The model under review builds one solid part; all positions refer to its coordinate system, in mm. Round coordinates to 2 decimals unless told otherwise and drop trailing zeros. Loops run counter-clockwise (first coordinate to the right, second up) from the corner with the lowest first, then second, coordinate; pieces in that order, holes last. Notation, with made-up numbers: (-2, 67.25) -> (21, 67.25) arc R16 cw to (21, 75.25) -> close; hole circle Ø10 at (39, 10.25). An arc over 180 degrees is marked (long way). Return JSON: item names as keys, results as strings. Group by question number.
```python
from build123d import *

# Parameters (mm, degrees)
F0_W     = 80.518
F0_H     = 499.999
F1_DEPTH = 6.35
F2_W     = 67.818
F2_H     = 6.35
F3_DEPTH = 6.35
F5_DEPTH = 6.35
F6_DEPTH = 6.35
F7_DEPTH = 6.35


# Not quite as in the source:
# - a feature names something its author has since deleted; it is built from what else it names


with BuildPart() as f1:
    # F0 (on Top) → F1 (new body)
    with BuildSketch(Plane.XY):
        with Locations((40.259, 230.6542872722)):
            Rectangle(F0_W, F0_H)
    extrude(amount=F1_DEPTH)

    # F2 (on face) → F3 (join)
    with BuildSketch(Plane(origin=(0, 0, 0), x_dir=(1, 0, 0), z_dir=(0, 0, -1))):
        Polygon((80.518, 19.3452127278), (74.168, 19.3452127278), (74.168, 12.9952127278), (74.168, -474.3037872722), (74.168, -480.6537872722), (80.518, -480.6537872722), align=None)
        Polygon((6.35, 19.3452127278), (0, 19.3452127278), (0, -480.6537872722), (6.35, -480.6537872722), (6.35, -474.3037872722), (6.35, 12.9952127278), align=None)
        with Locations((40.259, 16.1702127278)):
            Rectangle(F2_W, F2_H)
        with Locations((40.259, -477.4787872722)):
            Rectangle(F2_W, F2_H)
    extrude(amount=F3_DEPTH)

    # F4 (on face) → F5 (join)
    with BuildSketch(Plane(origin=(0, 0, 0), x_dir=(1, 0, 0), z_dir=(0, 0, -1))):
        Polygon((43.434, 12.9952127278), (37.084, 12.9952127278), (37.084, -7.4495371679), (37.084, -27.9419109224), (37.084, -69.0037844682), (37.084, -89.3237844682), (37.084, -130.4718448913), (37.084, -150.7918448913), (37.084, -191.9399053144), (37.084, -212.2599053144), (37.084, -253.4079657375), (37.084, -263.5679657375), (37.084, -273.7279657375), (37.084, -314.8760261606), (37.084, -335.1960261606), (37.084, -376.3440865837), (37.084, -386.5040865837), (37.084, -396.6640865837), (37.084, -437.8136164283), (37.084, -458.1321470068), (37.084, -474.3037872722), (43.434, -474.3037872722), (43.434, -457.6869668698), (43.434, -437.3826820421), (43.434, -396.2331521975), (43.434, -386.0731521975), (43.434, -375.9131521975), (43.434, -334.8512786517), (43.434, -314.3589048972), (43.434, -273.4694051058), (43.434, -263.2232182286), (43.434, -252.9770313513), (43.434, -212.08753156), (43.434, -191.5951578055), (43.434, -150.6912914171), (43.434, -130.2132842596), (43.434, -89.3237844682), (43.434, -68.8314107138), (43.434, -27.9419109224), (43.434, -7.5214582917), align=None)
        Polygon((48.5570884026, -319.4891816343), (43.434, -314.3589048972), (43.434, -334.8512786517), (48.5570884026, -329.7210019146), (74.168, -355.2960285474), (74.168, -345.1360285474), (53.6658303382, -324.6050917744), (74.168, -304.0741550015), (74.168, -293.9141550015), align=None)
        Polygon((48.5132602963, -442.4548254861), (43.434, -437.3826820421), (43.434, -457.6869668698), (48.5139950064, -452.6140897452), (70.2341258947, -474.3037872722), (74.168, -474.3037872722), (74.168, -468.0736188151), (53.5932553027, -447.5277026107), (74.168, -426.9240889705), (74.168, -416.7640889705), align=None)
        Polygon((37.084, -458.1321470068), (37.084, -437.8136164283), (32.0047397037, -442.8857598723), (6.35, -417.1950233567), (6.35, -427.3550233567), (26.9247446973, -447.9586369969), (6.35, -468.5045532013), (6.35, -474.3037872722), (10.7154131464, -474.3037872722), (32.0040049936, -453.0450241314), align=None)
        Polygon((6.35, -417.1950233567), (32.0040049936, -391.5769637083), (26.9240099873, -386.4898408329), (6.35, -407.0350233567), align=None)
        Polygon((53.5939900127, -386.0589064467), (48.5139950064, -391.1460293221), (74.168, -416.7640889705), (74.168, -406.6040889705), align=None)
        Polygon((48.5570884026, -196.7254345426), (43.434, -191.5951578055), (43.434, -212.08753156), (48.5570884026, -206.9572548229), (74.168, -232.5322814557), (74.168, -222.3722814557), (53.6658303382, -201.8413446827), (74.168, -181.3104079098), (74.168, -171.1504079098), align=None)
        Polygon((74.168, -232.5322814557), (48.5570884026, -258.1073080885), (53.6658303382, -263.2232182286), (74.168, -242.6922814557), align=None)
        Polygon((37.084, -335.1960261606), (37.084, -314.8760261606), (32.0040049936, -319.9489032852), (6.35, -294.2589025105), (6.35, -304.4189025105), (26.9240099873, -325.0217804098), (6.35, -345.5669629336), (6.35, -355.7269629336), (32.0040049936, -330.1089032852), align=None)
        Polygon((26.9240099873, -263.5537199867), (32.0040049936, -258.4808428621), (6.35, -232.7908420874), (6.35, -242.9508420874), align=None)
    extrude(amount=F5_DEPTH)

    # F4 (on face) → F6 (join)
    with BuildSketch(Plane(origin=(0, 0, 0), x_dir=(1, 0, 0), z_dir=(0, 0, -1))):
        Polygon((37.084, -150.7918448913), (37.084, -130.4718448913), (32.0040049936, -135.5447220159), (6.35, -109.8547212412), (6.35, -120.0147212412), (26.9240099873, -140.6175991405), (6.35, -161.1627816643), (6.35, -171.3227816643), (32.0040049936, -145.7047220159), align=None)
        Polygon((48.5570884026, -135.3435609967), (43.434, -130.2132842596), (43.434, -150.6912914171), (48.5570884026, -145.575381277), (74.168, -171.1504079098), (74.168, -160.9904079098), (53.6658303382, -140.4594711369), (74.168, -119.9285343639), (74.168, -109.7685343639), align=None)
        Polygon((31.9609115974, -12.579813905), (6.35, 12.9952127278), (6.35, 2.8352127278), (26.8521696618, -17.6957240451), (6.35, -38.2266608181), (6.35, -48.3866608181), (31.9609115974, -22.8116341853), (37.084, -27.9419109224), (37.084, -7.4495371679), align=None)
        Polygon((74.168, 2.8352127278), (74.168, 12.9952127278), (48.5211278761, -12.6157240451), (43.434, -7.5214582917), (43.434, -27.9419109224), (48.5570884026, -22.8116341853), (74.168, -48.3866608181), (74.168, -38.2266608181), (53.637083409, -17.7245113099), align=None)
        Polygon((48.5570884026, -73.9616874509), (43.434, -68.8314107138), (43.434, -89.3237844682), (48.5570884026, -84.1935077311), (74.168, -109.7685343639), (74.168, -99.6085343639), (53.6658303382, -79.077597591), (74.168, -58.5466608181), (74.168, -48.3866608181), align=None)
    extrude(amount=F6_DEPTH)

    # F4 (on face) → F7 (join)
    with BuildSketch(Plane(origin=(0, 0, 0), x_dir=(1, 0, 0), z_dir=(0, 0, -1))):
        Polygon((32.0040049936, -74.0766615928), (6.35, -48.3866608181), (6.35, -58.5466608181), (26.9240099873, -79.1495387174), (6.35, -99.6947212412), (6.35, -109.8547212412), (32.0040049936, -84.2366615928), (37.084, -89.3237844682), (37.084, -69.0037844682), align=None)
        Polygon((37.084, -212.2599053144), (37.084, -191.9399053144), (32.0040049936, -197.012782439), (6.35, -171.3227816643), (6.35, -181.4827816643), (26.9240099873, -202.0856595636), (6.35, -222.6308420874), (6.35, -232.7908420874), (32.0040049936, -207.172782439), align=None)
    extrude(amount=F7_DEPTH)


solid = f1.part
```
1. We need section A-A, the plane y = 273.5. Write out the cut boundary in (x, z).
2. Wall thickness on line 1 (X direction, y = 386, z = -5.5); line 2 (X direction, y = 423, z = -3); line 3 (X direction, y = 11.5, z = -1): over which ranges is each line inside the solid? List them lowest first.
3. We need section B-B, the plane y = 124.5. Write out the cut boundary in (x, z).
4. For P1, Ø6, axis at x = 12.5, y = 81.5, coming from the -Z side, flat-tipped, find the tip position at first contact; note if it passes through.
Check sheet entries:
{
 "1": {"outline": "(0, -6.35) -> (6.35, -6.35) -> (6.35, 0) -> (37.08, 0) -> (37.08, -6.35) -> (43.43, -6.35) -> (43.43, 0) -> (74.17, 0) -> (74.17, -6.35) -> (80.52, -6.35) -> (80.52, 6.35) -> (0, 6.35) -> close"},
 "2": {"line 1": "x = 0 to 6.35, 37.08 to 43.43, 74.17 to 80.52", "line 2": "x = 0 to 12.15, 37.08 to 43.43, 67.94 to 80.52", "line 3": "x = 0 to 6.35, 20.67 to 30.88, 33.04 to 47.41, 49.64 to 59.85, 74.17 to 80.52"},
 "3": {"outline": "(0, -6.35) -> (6.35, -6.35) -> (6.35, 0) -> (10.83, 0) -> (10.83, -6.35) -> (20.97, -6.35) -> (20.97, 0) -> (37.08, 0) -> (37.08, -6.35) -> (43.43, -6.35) -> (43.43, 0) -> (59.42, 0) -> (59.42, -6.35) -> (69.6, -6.35) -> (69.6, 0) -> (74.17, 0) -> (74.17, -6.35) -> (80.52, -6.35) -> (80.52, 6.35) -> (0, 6.35) -> close"},
 "4": {"P1": "stops at z = 0"}
}
